from build123d import *

# Parameters (mm, degrees)
F0_R            = 50
F0_R_2          = 13.5
F1_DEPTH        = 1.9
F3_DEPTH        = 25
F5_DEPTH        = 25
F5_COPIES_COUNT = 8


# Not quite as in the source:
# - a pattern or mirror of a feature is missing from the dataset's text; its kind, count and spacing are read off the source's solid


with BuildPart() as f1:
    # F0 (on Front) → F1 (new body)
    with BuildSketch(Plane.XZ):
        Circle(F0_R)
        Circle(F0_R_2, mode=Mode.SUBTRACT)
    extrude(amount=F1_DEPTH)

    # F2 (on Front) → F3 (cut)
    with BuildSketch(Plane.XZ):
        with BuildLine():
            Line((12.4794095755, 60.955286026), (0, 50.1961745322))
            Line((0, 50.1961745322), (2.7271706326, 35.8238514012))
            ThreePointArc((2.7271706326, 35.8238514012), (3.9364062163, 34.3449689954), (5.8350966322, 34.555488762))
            Line((5.8350966322, 34.555488762), (21.0234094411, 45.1330654323))
            Line((21.0234094411, 45.1330654323), (12.4794095755, 60.955286026))
        make_face()
    extrude(amount=-F3_DEPTH, mode=Mode.SUBTRACT)

    # F4 (on Front) → F5 (cut)
    with BuildSketch(Plane.XZ):
        with BuildLine():
            Line((10.4537707273, 34.3168952742), (22.7111335844, 48.0314604938))
            Line((22.7111335844, 48.0314604938), (18.2506803442, 59.0550513337))
            Line((18.2506803442, 59.0550513337), (1.7007282507, 51.2778109993))
            Line((1.7007282507, 51.2778109993), (1.0944613384, 48.079281378))
            Line((1.0944613384, 48.079281378), (7.1429279991, 34.8196319836))
            ThreePointArc((7.1429279991, 34.8196319836), (8.6623060706, 33.6723315481), (10.4537707273, 34.3168952742))
        make_face()
    f5 = extrude(amount=F5_DEPTH, mode=Mode.SUBTRACT)

    # F5_copies: F5 ×8 about axis
    f5_copies_axis = Axis((0, 0, 0), (0, 1, 0))
    for i in range(1, F5_COPIES_COUNT):
        add(f5.rotate(f5_copies_axis, i * 360 / F5_COPIES_COUNT), mode=Mode.SUBTRACT)


solid = f1.part
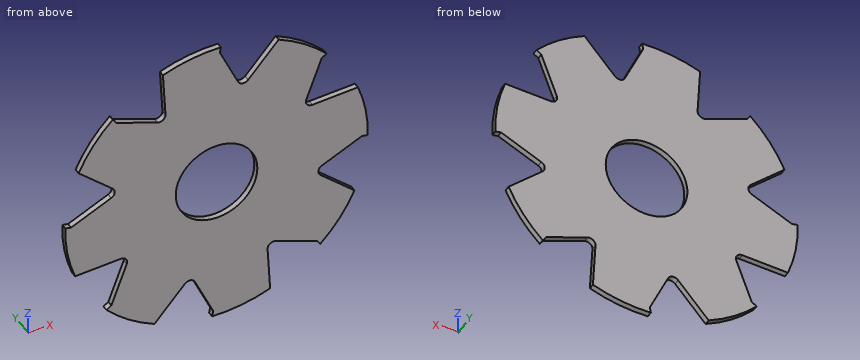
Verification items for the finished model (mm, model axes). Give positions to 0.01 mm unless a question says otherwise; leave off trailing zeros. Loops run counter-clockwise (first coordinate to the right, second up) from the corner with the lowest first, then second, coordinate; pieces in that order, holes last. Notation, with made-up numbers: (80.25, 8) - (100.25, 8) arc R21 cw to (100.25, 13) - close; hole circle Ø8 at (53, 64). An arc over 180 degrees is marked (long way). Write each question's results on one line, items separated by ' | '.
1) Material ranges on L1, parallel to Z at x = 0, y = -0.5; L2, parallel to X at y = -0.65, z = 5; L3, parallel to X at y = -0.4, z = 1.5, recorded low to high. Write a range as from..to.
Solution:
L1: -50..-13.5, 13.5..50 | L2: -39.52..-12.54, 12.54..49.75 | L3: -47.19..-13.42, 13.42..49.98
2) Sectioned sample at C-C on z = 28. Record the boundary of the cut face in (x, y), plus the area to 3 significant figures.
Solution:
outline: (-41.42, -1.9) - (32.82, -1.9) - (32.82, 0) - (-41.42, 0) - close | area: 141 mm2
3) Sectioned sample at A-A on x = -40. Record the boundary of the cut face in (y, z).
Solution:
outline: (-1.9, -17.34) - (0, -17.34) - (0, 4.78) - (-1.9, 4.78) - close; (-1.9, 15.53) - (0, 15.53) - (0, 30) - (-1.9, 30) - close
4) Depth check by flat-ended pin: P1, Ø2, axis at x = 9, z = 8.5, coming from the -Y side. Enter the tip coordinate at first touch or a pass-through.
Solution:
P1: through
5) Sectioned sample at B-B on z = -41. Record the boundary of the cut face in (x, y).
Solution:
outline: (-28.62, -1.9) - (-16.43, -1.9) - (-16.43, 0) - (-28.62, 0) - close; (-4.32, -1.9) - (17.4, -1.9) - (17.4, 0) - (-4.32, 0) - close
